Geometry: final body of the model. Coordinates: model frame, mm. Face numbers are marked on the shaded views. A direction names the side the tool comes from. Round coordinates to 2 decimals unless told otherwise and drop trailing zeros. Loops run counter-clockwise (first coordinate to the right, second up) from the corner with the lowest first, then second, coordinate; pieces in that order, holes last. Notation, with made-up numbers: M 14,-32.75 L 58,-32.75 A5 cw 58,-28.75 Z; hole C 72,-9 d3. An arc over 180 degrees is marked long. Write each question's results on one line, items separated by ' | '.
```python
from build123d import *

# Parameters (mm, degrees)
F0_R          = 10
F0_R_2        = 1.65
F1_DEPTH      = 7
F2_R          = 1.75
F3_DEPTH      = 25
F3_DEPTH_BACK = 5


with BuildPart() as f1:
    # F0 (on Top) → F1 (new body)
    with BuildSketch(Plane.XY):
        Circle(F0_R)
        with Locations((0, -7)):
            Circle(F0_R_2, mode=Mode.SUBTRACT)
        Polygon((-0.2828427125, -3.8183766184), (1.767766953, -1.767766953), (3.8183766184, 0.2828427125), (5.939696962, -1.8384776311), (1.8384776311, -5.939696962), align=None, mode=Mode.SUBTRACT)
        with Locations((-7, 0)):
            Circle(F0_R_2, mode=Mode.SUBTRACT)
        with BuildLine():
            ThreePointArc((1.166726189, -1.166726189), (-1.5244012286, 0.6314276634), (1.65, 0))
            ThreePointArc((1.65, 0), (1.5244012286, -0.6314276634), (1.166726189, -1.166726189))
        make_face(mode=Mode.SUBTRACT)
        with Locations((7, 0)):
            Circle(F0_R_2, mode=Mode.SUBTRACT)
        with Locations((0, 7)):
            Circle(F0_R_2, mode=Mode.SUBTRACT)
    extrude(amount=F1_DEPTH)

    # F2 (on face) → F3 (cut, two sides)
    with BuildSketch(Plane(origin=(3.8890872965, -3.8890872965, 0), x_dir=(-0.7071067812, -0.7071067812, 0), z_dir=(-0.7071067812, 0.7071067812, 0))) as f3_sk:
        with Locations((0, 3.5)):
            Circle(F2_R)
    extrude(amount=-F3_DEPTH, mode=Mode.SUBTRACT)
    extrude(f3_sk.sketch, amount=F3_DEPTH_BACK, mode=Mode.SUBTRACT)


solid = f1.part
```
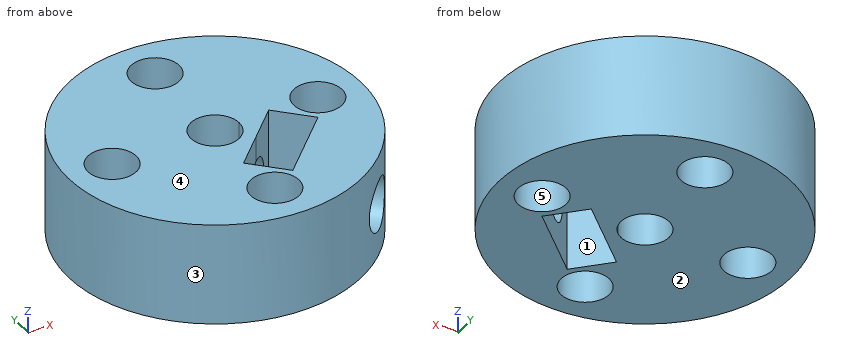
1. Section B-B (x = -7). Output: boundary loops of the cut face in (y, z).
Answer key:
outline: M -7.14,0 L -1.65,0 L -1.65,7 L -7.14,7 Z; M 1.65,0 L 7.14,0 L 7.14,7 L 1.65,7 Z
2. Ray query, probe 1 along X at (y, z) = (-1.5, 4.25); probe 2 along X at (y, z) = (1, 6.25); probe 3 along Y at (x, z) = (-7.75, 5). Return the intervals inside material, ascending.
Answer key:
probe 1: x = -9.89 to -7.69, -6.31 to -0.74, 5.6 to 6.31, 7.69 to 9.89 | probe 2: x = -9.95 to -8.31, -5.69 to -1.31, 1.31 to 5.69, 8.31 to 9.95 | probe 3: y = -6.32 to -1.47, 1.47 to 6.32
3. Draft query along X for the marked faces 3, 4 and 5. Return one class per face: pulls with the +X half, pulls with the -X half, needs draft (parallel to the pull), parting line crosses it, or undercut.
Answer key:
face 3: parting line crosses it | face 4: needs draft | face 5: undercut
4. Section D-D (z = 3.75). Output: boundary loops of the cut face in (x, y).
Answer key:
outline: M -0.87,-1.58 L -0.76,-1.47 A1.65 cw long 1.47,0.76 L 1.58,0.87 L 2.99,-0.54 L 3.82,0.28 L 5.94,-1.84 L 5.11,-2.66 L 8.19,-5.74 A10 ccw long 5.74,-8.19 L 2.66,-5.11 L 1.84,-5.94 L -0.28,-3.82 L 0.54,-2.99 Z; hole C -7,0 d3.3; hole C 0,-7 d3.3; hole C 0,7 d3.3; hole C 7,0 d3.3
5. Access query for the marked faces 1 and 2. Directions: +Z, -Z, +X, -X, +Y, -Y. A direction counts if a zero-diameter tool reaches every point of the face in a straight line with its end or side. Return the directions, or none.
Answer key:
face 1: +Z, -Z | face 2: -Z, +X, -X, +Y, -Y
6. Section A-A (z = 5.75). Output: boundary loops of the cut face in (x, y).
Answer key:
outline: C 0,0 d20; hole C -7,0 d3.3; hole C 0,-7 d3.3; hole C 0,0 d3.3; hole C 0,7 d3.3; hole M -0.28,-3.82 L 1.84,-5.94 L 5.94,-1.84 L 3.82,0.28 Z; hole C 7,0 d3.3
7. Pin query (flat end, axial travel): P1, Ø1, axis at y = 3, z = 5, coming from the +X side; P2, Ø2, axis at x = 0, y = -7, coming from the -Z side; P3, Ø3, axis at y = -6.5, z = 1, coming from the -X side. Return the tip coordinate at first contact, or that it passes through.
Answer key:
P1: stops at x = 9.68 | P2: passes through | P3: stops at x = -8.66
